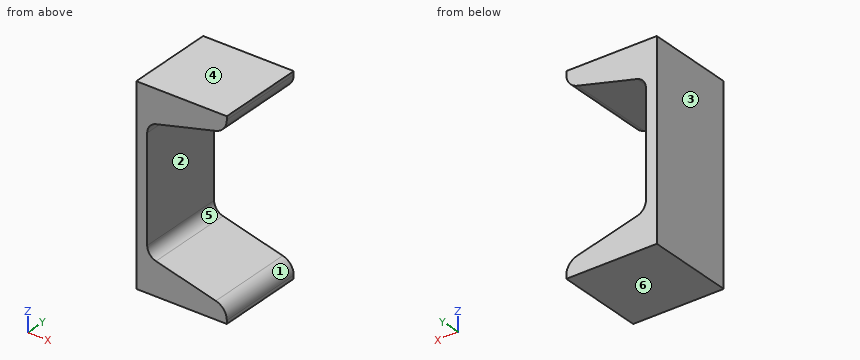
Solid Edge part; units mm, degrees
sketch "Sketch1" plane through (0, 0, 0) normal (0, -1, 0) x (1, 0, 0)
  line L0 (0, 38.1) -> (35.814, 38.1)
  line L1 (35.814, 38.1) -> (35.814, 36.7644)
  arc A0 (35.814, 36.7644) -> (31.4663, 31.1658) centre (30.0355, 36.7644) cw
  line L2 (31.4663, 31.1658) -> (7.7961, 25.1163)
  arc A1 (7.7961, 25.1163) -> (4.318, 20.6375) centre (8.9408, 20.6375) ccw
  line L3 (4.318, -20.6375) -> (4.318, 20.6375)
  arc A2 (7.7961, -25.1163) -> (4.318, -20.6375) centre (8.9408, -20.6375) cw
  line L4 (31.4663, -31.1658) -> (7.7961, -25.1163)
  arc A3 (35.814, -36.7644) -> (31.4663, -31.1658) centre (30.0355, -36.7644) ccw
  line L5 (35.814, -38.1) -> (35.814, -36.7644)
  line L6 (0, -38.1) -> (35.814, -38.1)
  line L7 (0, 38.1) -> (0, -38.1)
extrude "Protrusion1" add sketch "Sketch1" against normal blind 34.925
Input: part model. Units: mm. Frame: model coordinates. Face numbers are marked on the shaded views. A direction names the side the tool comes from. Give positions to 0.01 mm unless a question says otherwise; leave off trailing zeros. Order: outer loops, then holes, each group sorted by start corner. A loop starts at its lowest first (then second) coordinate and runs counter-clockwise, first axis right, second up.
Q1. Section C-C on z = -1.5. Output: boundary loops of the cut face in (x, y) (3 decimals), and give its area (3 significant figures).
Checked values:
outline: (0, 0) - (4.318, 0) - (4.318, 34.925) - (0, 34.925) - close
area: 151 mm2
Q2. Draft query along Z for the marked faces 1, 2, 3 and 4. Return one class per face: +Z half, -Z half, draft (parallel to the pull), parting line (faces both ways), or undercut.
Checked values:
face 1: undercut
face 2: undercut
face 3: draft
face 4: +Z half
Q3. Section A-A on x = 12. Output: boundary loops of the cut face in (y, z) (3 decimals), and give its area (3 significant figures).
Checked values:
outline: (0, -38.1) - (34.925, -38.1) - (34.925, -26.191) - (0, -26.191) - close; (0, 26.191) - (34.925, 26.191) - (34.925, 38.1) - (0, 38.1) - close
area: 832 mm2
Q4. Ray query, probe 1 along X at (y, z) = (12, -4); probe 2 along Z at (x, y) = (30, 32); probe 3 along Z at (x, y) = (17, 24). Return the intervals inside material, ascending.
Checked values:
probe 1: x = 0 to 4.32
probe 2: z = -38.1 to -30.79, 30.79 to 38.1
probe 3: z = -38.1 to -27.47, 27.47 to 38.1
Q5. Section B-B on y = 27. Output: boundary loops of the cut face in (x, z).
Checked values:
outline: (0, -38.1) - (35.81, -38.1) - (35.81, -36.76) arc R5.78 ccw to (31.47, -31.17) - (7.8, -25.12) arc R4.62 cw to (4.32, -20.64) - (4.32, 20.64) arc R4.62 cw to (7.8, 25.12) - (31.47, 31.17) arc R5.78 ccw to (35.81, 36.76) - (35.81, 38.1) - (0, 38.1) - close
Q6. Section D-D on x = 5.5. Output: boundary loops of the cut face in (y, z) (3 decimals), and give its area (3 significant figures).
Checked values:
outline: (0, -38.1) - (34.925, -38.1) - (34.925, -23.725) - (0, -23.725) - close; (0, 23.725) - (34.925, 23.725) - (34.925, 38.1) - (0, 38.1) - close
area: 1,000 mm2
Q7. Set-up query: the marked faces 5 and 6. Return all of +Z, -Z, +X, -X, +Y, -Y with unobstructed straight access to the full face (end or side cutting, diameter ignored); none if empty.
Checked values:
face 5: +X, +Y, -Y
face 6: -Z, +X, -X, +Y, -Y
